For this review, take the finished solid that the model builds, in its own axes (mm). Face numbers are marked on the shaded views. Coordinates: 2 decimals unless noted, no trailing zeros. Loops run counter-clockwise (first coordinate to the right, second up) from the corner with the lowest first, then second, coordinate; pieces in that order, holes last.
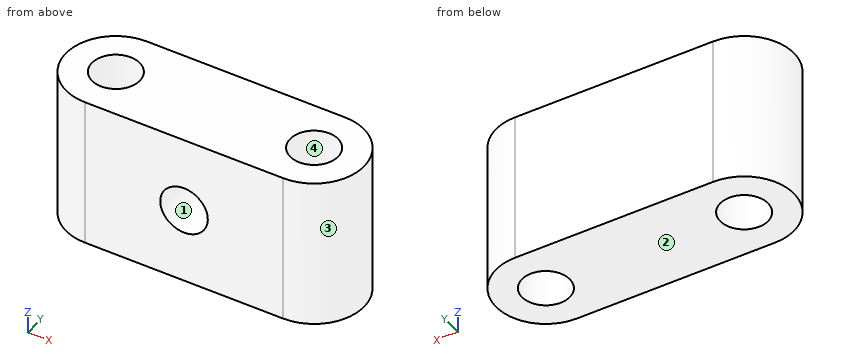
```python
from build123d import *

# Parameters (mm, degrees)
SKETCH1_R           = 6
BOSS_EXTRUDE1_DEPTH = 19
SKETCH2_R           = 6
CUT_EXTRUDE1_DEPTH  = 12.5


with BuildPart() as part:
    # Sketch1 → Boss-Extrude1 (new, symmetric)
    with BuildSketch(Plane.XY):
        with BuildLine():
            Line((0, 12.5), (50, 12.5))
            ThreePointArc((50, 12.5), (62.5, 0), (50, -12.5))
            Line((50, -12.5), (0, -12.5))
            ThreePointArc((0, -12.5), (-12.5, 0), (0, 12.5))
        make_face()
        Circle(SKETCH1_R, mode=Mode.SUBTRACT)
        with Locations((50, 0)):
            Circle(SKETCH1_R, mode=Mode.SUBTRACT)
    extrude(amount=BOSS_EXTRUDE1_DEPTH, both=True)

    # Sketch2 → Cut-Extrude1 (cut)
    with BuildSketch(Plane.XZ.offset(12.5)):
        with Locations(Location((25, 0, 0), (0, 0, 270))):
            Circle(SKETCH2_R)
    extrude(amount=-CUT_EXTRUDE1_DEPTH, mode=Mode.SUBTRACT)


solid = part.part
```
Q1. Wall thickness on probe 1 along X at (y, z) = (5, 14); probe 2 along X at (y, z) = (-0.5, -13.5); probe 3 along X at (y, z) = (-1.75, 0.5): over which ranges is each line inside the solid? List them lowest first.
Q2. Consider section C-C (x = -1.5). State the section outline as (y, z) points.
Q3. For pin 1 Ø6 at (x, z) = (24, -2) entering from -Y; pin 2 Ø8 at (y, z) = (5.5, -10) entering from -X; pin 3 Ø1 at (y, z) = (-5.5, 10.5) entering from -X; pin 4 Ø7 at (x, y) = (50, 0) entering from -Z, all flat-tipped, find the tip position at first contact; note any pin that passes through.
Q4. Consider section A-A (z = 0). State the section outline as (x, y) points, then the cut area to 3 significant figures.
Q5. The part is to be moulded in two halves that separate along X. For the marked faces 1, 2, 3 and 4, say which applies: +X half, -X half, draft (parallel to the pull), parting line (faces both ways), or undercut.
Q6. Consider section D-D (z = 8). State the section outline as (x, y) points, then the cut area to 3 significant figures.
Q7. Consider section B-B (x = 25). State the section outline as (y, z) points, then the cut area to 3 significant figures.
Model answer:
1. probe 1: x = -11.46 to -3.32, 3.32 to 46.68, 53.32 to 61.46
1. probe 2: x = -12.49 to -5.98, 5.98 to 44.02, 55.98 to 62.49
1. probe 3: x = -12.38 to -5.74, 5.74 to 19.02, 30.98 to 44.26, 55.74 to 62.38
2. outline: (-12.41, -19) - (-5.81, -19) - (-5.81, 19) - (-12.41, 19) - close; (5.81, -19) - (12.41, -19) - (12.41, 19) - (5.81, 19) - close
3. pin 1: stops at y = 0
3. pin 2: stops at x = -12.41
3. pin 3: stops at x = -11.46
3. pin 4: passes through
4. outline: (0, -12.5) - (19, -12.5) - (19, 0) - (31, 0) - (31, -12.5) - (50, -12.5) arc R12.5 ccw to (50, 12.5) - (0, 12.5) arc R12.5 ccw to start; hole circle Ø12 at (0, 0); hole circle Ø12 at (50, 0)
4. area: 1,360 mm2
5. face 1: undercut
5. face 2: draft
5. face 3: +X half
5. face 4: undercut
6. outline: (0, -12.5) - (50, -12.5) arc R12.5 ccw to (50, 12.5) - (0, 12.5) arc R12.5 ccw to start; hole circle Ø12 at (0, 0); hole circle Ø12 at (50, 0)
6. area: 1,510 mm2
7. outline: (-12.5, -19) - (12.5, -19) - (12.5, 19) - (-12.5, 19) - (-12.5, 6) - (0, 6) - (0, -6) - (-12.5, -6) - close
7. area: 800 mm2
